Input: part model. Units: mm. Frame: model coordinates. A direction names the side the tool comes from. Give positions to 0.01 mm unless a question says otherwise; leave off trailing zeros. Loops run counter-clockwise (first coordinate to the right, second up) from the corner with the lowest first, then second, coordinate; pieces in that order, holes last. Notation, with made-up numbers: M -12.5,50.5 L -1.5,50.5 A30 cw -1.5,77.5 Z; hole C 13,-34.5 d5. An arc over 180 degrees is marked long. Answer as a JSON object with one key per item and string values. Group by question number.
1) Section query C-C on y = -20. Return loops of the section in (x, z), plus the area to 3 significant figures.
2) Ray query, L1, parallel to X at y = -31, z = 28; L2, parallel to Y at x = 58.5, z = 42; L3, parallel to Z at x = 16, y = -8. Return the intervals inside material, ascending.
3) Section query D-D on z = 40. Return loops of the section in (x, y).
4) Draft query along X for faces 3 (the flat face through (62.397, -16, 31)), 4 (the flat face through (-7.453, -16, 25)), 5 (the flat face through (30, 9.35, 25)). Return one class per face: +X half, -X half, draft (parallel to the pull), parting line (faces both ways), or undercut.
5) Section query A-A on z = 16. Return loops of the section in (x, y), plus the area to 3 significant figures.
6) Section query B-B on x = 22.5. Return loops of the section in (y, z).
7) First-contact query: P1, Ø5, axis at x = 32.08, y = -14.58, coming from the +Z side; P2, Ø1.8, axis at x = 30.5, y = -39.5, coming from the +Z side; P3, Ø5, axis at x = 7.5, y = -32, coming from the +Z side. Flat tips, straight axial feed; report the tip coordinate or a pass-through.
8) Access query for faces 1 (the flat face through (31, 7, 38.1)), 2 (the cylindrical face through (33.783, -11.907, 5.151)). Directions: +Z, -Z, +X, -X, +Y, -Y. A direction counts if a zero-diameter tool reaches every point of the face in a straight line with its end or side. Return the directions, or none.
from build123d import *

# Parameters (mm, degrees)
SKETCH9_W           = 76.2
SKETCH9_H           = 50.8
BOSS_EXTRUDE2_DEPTH = 50.8
SKETCH10_W          = 63.5
SKETCH10_H          = 20.32
CUT_EXTRUDE3_DEPTH  = 40.64
SKETCH11_R          = 1.5875
SKETCH11_R_2        = 3.175
CUT_EXTRUDE4_DEPTH  = 90.976761381
SKETCH12_R          = 1.778
CUT_EXTRUDE5_DEPTH  = 12.7
SKETCH19_R          = 1.778
CUT_EXTRUDE9_DEPTH  = 12.7


with BuildPart() as part:
    # Sketch9 → Boss-Extrude2 (new body)
    with BuildSketch(Plane.XY):
        with Locations((30.646725964, -16.049917464)):
            Rectangle(SKETCH9_W, SKETCH9_H)
    extrude(amount=BOSS_EXTRUDE2_DEPTH)

    # Sketch10 → Cut-Extrude3 (cut)
    with BuildSketch(Plane.XY.offset(50.8)):
        with Locations((30.646725964, -5.889917464)):
            Rectangle(SKETCH10_W, SKETCH10_H)
        with Locations((30.646725964, -26.209917464)):
            Rectangle(SKETCH10_W, SKETCH10_H)
    extrude(amount=-CUT_EXTRUDE3_DEPTH, mode=Mode.SUBTRACT)

    # Sketch11 → Cut-Extrude4 (cut, through all)
    with BuildSketch(Plane.XY.offset(10.16)):
        with Locations((15.566258562, -14.584417496)):
            Circle(SKETCH11_R)
        with Locations((32.076258562, -14.584417496)):
            Circle(SKETCH11_R_2)
    extrude(amount=-CUT_EXTRUDE4_DEPTH, mode=Mode.SUBTRACT)

    # Sketch12 → Cut-Extrude5 (cut)
    with BuildSketch(Plane.XY.offset(50.8)):
        with Locations((30.646725964, 6.810082536)):
            Circle(SKETCH12_R)
    extrude(amount=-CUT_EXTRUDE5_DEPTH, mode=Mode.SUBTRACT)

    # Sketch19 → Cut-Extrude9 (cut)
    with BuildSketch(Plane.XY.offset(50.8)):
        with Locations((30.627843478, -39.011499114)):
            Circle(SKETCH19_R)
    extrude(amount=-CUT_EXTRUDE9_DEPTH, mode=Mode.SUBTRACT)


solid = part.part
Output:
{
 "1": {"outline": "M -7.45,0 L 68.75,0 L 68.75,50.8 L 62.4,50.8 L 62.4,10.16 L -1.1,10.16 L -1.1,50.8 L -7.45,50.8 Z", "area": "1,290 mm^2"},
 "2": {"L1": "x = -7.45 to -1.1, 62.4 to 68.75", "L2": "y = -41.45 to -36.37, 4.27 to 9.35", "L3": "z = 0 to 10.16"},
 "3": {"outline": "M -7.45,-41.45 L 68.75,-41.45 L 68.75,9.35 L -7.45,9.35 Z; hole M -1.1,-36.37 L 62.4,-36.37 L 62.4,4.27 L -1.1,4.27 Z; hole C 30.63,-39.01 d3.56; hole C 30.65,6.81 d3.56"},
 "4": {"face 3": "undercut", "face 4": "-X half", "face 5": "draft"},
 "5": {"outline": "M -7.45,-41.45 L 68.75,-41.45 L 68.75,9.35 L -7.45,9.35 Z; hole M -1.1,-36.37 L 62.4,-36.37 L 62.4,4.27 L -1.1,4.27 Z", "area": "1,290 mm^2"},
 "6": {"outline": "M -41.45,0 L 9.35,0 L 9.35,50.8 L 4.27,50.8 L 4.27,10.16 L -36.37,10.16 L -36.37,50.8 L -41.45,50.8 Z"},
 "7": {"P1": "passes through", "P2": "stops at z = 38.1", "P3": "stops at z = 10.16"},
 "8": {"face 1": "+Z", "face 2": "+Z, -Z"}
}
